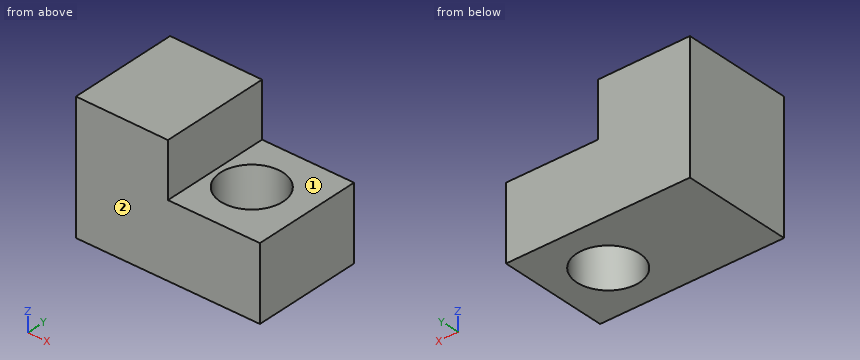
```python
from build123d import *

# Parameters (mm, degrees)
F1_DEPTH = 762
F2_R     = 215.9
F3_DEPTH = 508.001


with BuildPart() as f1:
    # F0 (on Front) → F1 (new body)
    with BuildSketch(Plane.XZ):
        Polygon((579.295597, 110.950105), (-55.692269, 114.875649), (-55.692269, -774.124351), (1214.307731, -774.124351), (1214.307731, -266.124351), (579.295597, -266.124351), align=None)
    extrude(amount=F1_DEPTH)

    # F2 (on face) → F3 (cut, through all)
    with BuildSketch(Plane.XY.offset(-266.124351)):
        with Locations((833.307731, -381)):
            Circle(F2_R)
    extrude(amount=-F3_DEPTH, mode=Mode.SUBTRACT)


solid = f1.part
```
The listing builds one solid part. Answer for the finished solid, in the listing's coordinates (mm). Face numbers are marked on the shaded views. A direction names the side the tool comes from. Coordinates: 2 decimals unless noted, no trailing zeros. Loops run counter-clockwise (first coordinate to the right, second up) from the corner with the lowest first, then second, coordinate; pieces in that order, holes last. Notation, with made-up numbers: (31, 84.5) - (55, 84.5) arc R10 ccw to (55, 99.5) - close; hole circle Ø4 at (-6.75, 52.25). An arc over 180 degrees is marked (long way). Use a Markdown table: item, result. Add a question column.
1) Find the intervals of material crossed by line 1 (X direction, y = -346.5, z = -711); line 2 (Z direction, x = 580.5, y = -210); line 3 (Y direction, x = 745.5, z = -407), in increasing order.
2) The part is cut by section A-A, the plane y = -381. Give the vertices of the cut face in (x, z).
3) For the marked faces 1 and 2, determine the directions among +Z, -Z, +X, -X, +Y, -Y from which every point of the face is accessible in a straight line to the end or side of a thin tool.
4) Given pin 1 (2 mm diameter, centred on y = -643.5, z = -264, fed in from +X), flat-ended and moving along its own axis, determine where the tip first touches the part or whether it passes through.
5) The part is cut by section B-B, the plane x = 761. Give the vertices of the cut face in (y, z), and give its area (3 significant figures).
6) The part is cut by section D-D, the plane y = -682. Give the vertices of the cut face in (x, z), and give its area (3 significant figures).
7) The part is cut by section C-C, the plane z = -370.5. Give the vertices of the cut face in (x, y).
Here are the results:
| question | item | result |
|---|---|---|
| 1 | line 1 | x = -55.69 to 620.18, 1046.43 to 1214.31 |
| 1 | line 2 | z = -774.12 to -266.12 |
| 1 | line 3 | y = -762 to -578.24, -183.76 to 0 |
| 2 | outline | (-55.69, -774.12) - (617.41, -774.12) - (617.41, -266.12) - (579.3, -266.12) - (579.3, 110.95) - (-55.69, 114.88) - close; (1049.21, -774.12) - (1214.31, -774.12) - (1214.31, -266.12) - (1049.21, -266.12) - close |
| 3 | face 1 | +Z, +X, +Y, -Y |
| 3 | face 2 | +Z, -Z, +X, -X, -Y |
| 4 | pin 1 | stops at x = 579.3 |
| 5 | outline | (-762, -774.12) - (-584.43, -774.12) - (-584.43, -266.12) - (-762, -266.12) - close; (-177.57, -774.12) - (0, -774.12) - (0, -266.12) - (-177.57, -266.12) - close |
| 5 | area | 180,000 mm^2 |
| 6 | outline | (-55.69, -774.12) - (1214.31, -774.12) - (1214.31, -266.12) - (579.3, -266.12) - (579.3, 110.95) - (-55.69, 114.88) - close |
| 6 | area | 886,000 mm^2 |
| 7 | outline | (-55.69, -762) - (1214.31, -762) - (1214.31, 0) - (-55.69, 0) - close; hole circle Ø431.8 at (833.31, -381) |
